```python
from build123d import *

# Parameters (mm, degrees)
BOSS_EXTRUDE1_DEPTH      = 3.175
F_1_0_1_DIAMETER_HOLE1_D = 3
F_3_0_3_DIAMETER_HOLE1_D = 3


with BuildPart() as part:
    # Sketch1 → Boss-Extrude1 (new body)
    with BuildSketch(Plane(origin=(0, 0, 0), x_dir=(1, 0, 0), z_dir=(0, 1, 0))):
        Polygon((0, 190), (-3.175, 190), (-3.175, 150), (0, 150), (0, 50), (-3.175, 50), (-3.175, 10), (0, 10), (0, 0), (156.24, 0), (156.24, 10), (159.415, 10), (159.415, 50), (156.24, 50), (156.24, 150), (159.415, 150), (159.415, 190), (156.24, 190), (156.24, 200), (0, 200), align=None)
    extrude(amount=BOSS_EXTRUDE1_DEPTH)

    # Ø1.0 (1) Diameter Hole1 (through all)
    with Locations(Plane(origin=(0, 3.175, 0), x_dir=(1, 0, 0), z_dir=(0, 1, 0))):
        with Locations((47.327548064, 144.467472705), (6.682102799, 144.467472705), (57.426953427, 168.726839726), (83.629599498, 190.400856446), (108.822249068, 144.454220349), (149.551998107, 144.454220349), (47.417498943, 55.54499618), (108.822508358, 55.54499618), (149.552467088, 55.54499618), (71.619997678, 21.799999041), (6.6874813, 55.54499618)):
            Hole(F_1_0_1_DIAMETER_HOLE1_D / 2)

    # Ø3.0 (3) Diameter Hole1 (through all)
    with Locations(Plane(origin=(0, 3.175, 0), x_dir=(1, 0, 0), z_dir=(0, 1, 0))):
        with Locations((63.121282677, 131.000354826), (93.119995544, 130.999996355), (63.121282677, 71.000354826), (93.119995544, 70.999996355)):
            Hole(F_3_0_3_DIAMETER_HOLE1_D / 2)


solid = part.part
```
The listing builds one solid part. Answer for the finished solid, in the listing's coordinates (mm). Give positions to 0.01 mm unless a question says otherwise; leave off trailing zeros. Write each loop counter-clockwise with the first axis right and the second up, starting at its lowest first coordinate (ties: lowest second). Pieces come first, ordered by that corner, then holes. Notation, with made-up numbers: (19, 72.5) - (72, 72.5) arc R29 ccw to (72, 97.5) - close; hole circle Ø4 at (30, -7.5). An arc over 180 degrees is marked (long way). Use one line per item in the form item = value. Start each with the question number.
1) Flat-ended cylindrical pins translate along their axes: pin 1 Ø1.8 at (x, z) = (83.63, -190.4) entering from +Y; pin 2 Ø1.5 at (y, z) = (0.5, -131.5) entering from +X; pin 3 Ø1.6 at (x, y) = (158, 2) entering from -Z; pin 4 Ø1 at (x, y) = (-1.5, 2) entering from +Z. Find the tip coordinate at first contact, or state that the pin passes through.
2) Find section A-A on z = -66. Determine the outline of the cut face in (x, y) (3 decimals), plus the area to 3 significant figures.
3) Consider line 1 along Z through (x, y) = (7, 1.6); line 2 along X through (y, z) = (1, -141). Determine where each line is inside the solid, lowest interval first. Write a range as from..to.
4) Find section B-B on y = 2.5. Count the separate pieces of the cut face and the enclosed holes in it, plus the area to 4 significant figures.
Geometry results:
q1.pin_1 = through
q1.pin_2 = 156.24
q1.pin_3 = -190
q1.pin_4 = -10
q2.outline = (0, 0) - (156.24, 0) - (156.24, 3.175) - (0, 3.175) - close
q2.area = 496 mm2
q3.line_1 = -200..-145.93, -143..-57.01, -54.08..0
q3.line_2 = 0..156.24
q4.separate_pieces = 1
q4.enclosed_holes = 15
q4.area = 31,650 mm2
